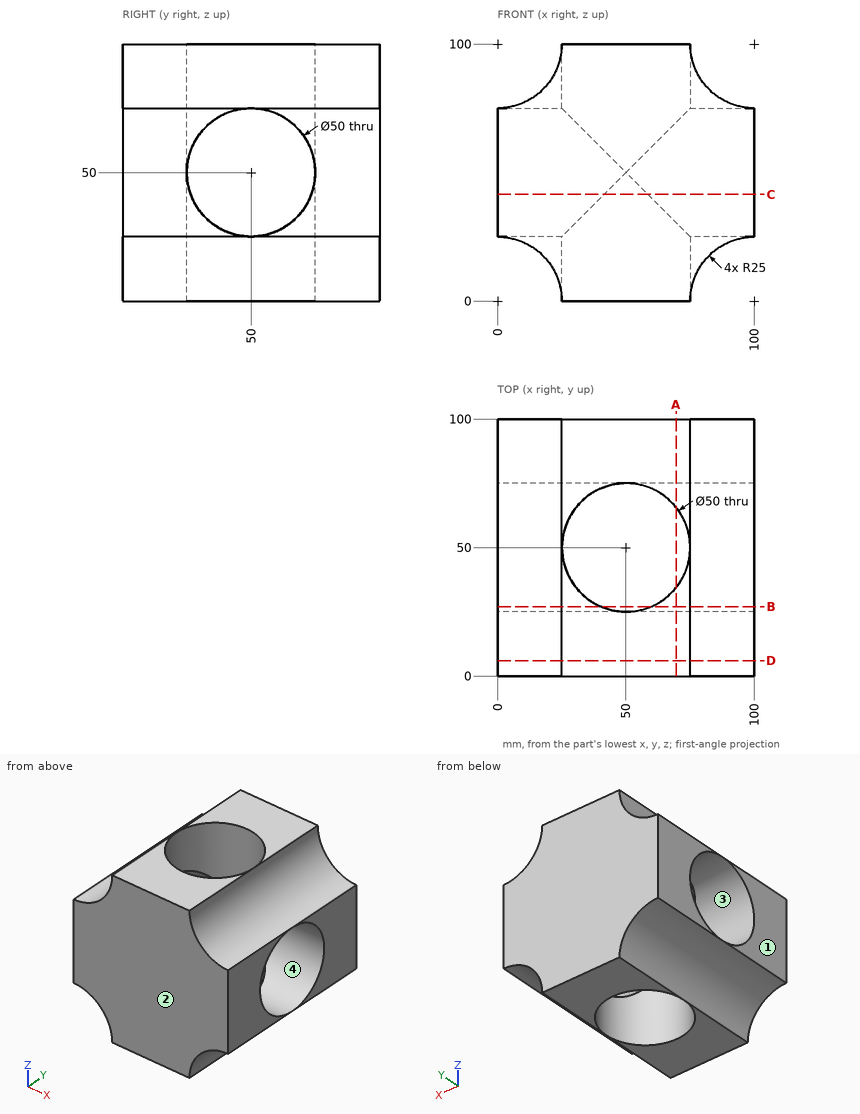
Here's the drawing with two shaded views (mm, measured from the low corner). I have some questions. Give positions to 0.01 mm unless a question says otherwise; leave off trailing zeros. Loops run counter-clockwise (first coordinate to the right, second up) from the corner with the lowest first, then second, coordinate; pieces in that order, holes last. Notation, with made-up numbers: (25.25, 73) -> (81.25, 73) arc R30 ccw to (81.25, 99) -> close; hole circle Ø4 at (72.5, -19.5). An arc over 180 degrees is marked (long way). Answer as a JSON object with one key per item and string values. Group by question number.
Item 1: Imagine slicing it at B-B on y = 27. Write out the boundary of the cut face in (x, z), then the cut area to 3 significant figures.
Item 2: Imagine slicing it at D-D on y = 6. Write out the boundary of the cut face in (x, z), then the cut area to 3 significant figures.
Item 3: Imagine slicing it at C-C on z = 41.5. Write out the boundary of the cut face in (x, y).
Item 4: Thinking about a two-plate mould opening in Y: for the marked faces 1, 2, 3 and 4, which applies, pulls with the +Y half, pulls with the -Y half, needs draft (parallel to the pull), parting line crosses it, or undercut?
Item 5: Imagine slicing it at A-A on x = 69.5. Write out the boundary of the cut face in (y, z), then the cut area to 3 significant figures.
Item 6: Will these pins go through, and if not, where does the flat tip stop? pin 1 (1 mm diameter, centred on x = 14.5, y = 30, fed in from +Z); pin 2 (8 mm diameter, centred on y = 71, z = 87.5, fed in from -X); pin 3 (1.5 mm diameter, centred on x = 13, y = 15.5, fed in from +Z).
Item 7: I need wall thicknesses on L1, parallel to Y at x = 13, z = 50; L2, parallel to Y at x = 77.5, z = 32.5; L3, parallel to X at y = 55, z = 78. Which ranges of each line are inside material? Lowest first, please.
Answer list:
{
 "1": {"outline": "(0, 25) arc R25 cw to (25, 0) -> (40.2, 0) -> (40.2, 40.2) -> (0, 40.2) -> close; (0, 59.8) -> (40.2, 59.8) -> (40.2, 100) -> (25, 100) arc R25 cw to (0, 75) -> close; (59.8, 0) -> (75, 0) arc R25 cw to (100, 25) -> (100, 40.2) -> (59.8, 40.2) -> close; (59.8, 59.8) -> (100, 59.8) -> (100, 75) arc R25 cw to (75, 100) -> (59.8, 100) -> close", "area": "4,500 mm2"},
 "2": {"outline": "(0, 25) arc R25 cw to (25, 0) -> (75, 0) arc R25 cw to (100, 25) -> (100, 75) arc R25 cw to (75, 100) -> (25, 100) arc R25 cw to (0, 75) -> close", "area": "8,040 mm2"},
 "3": {"outline": "(0, 0) -> (100, 0) -> (100, 26.49) -> (58.5, 26.49) arc R25 cw to (41.5, 26.49) -> (0, 26.49) -> close; (0, 73.51) -> (41.5, 73.51) arc R25 cw to (58.5, 73.51) -> (100, 73.51) -> (100, 100) -> (0, 100) -> close"},
 "4": {"face 1": "needs draft", "face 2": "pulls with the -Y half", "face 3": "undercut", "face 4": "undercut"},
 "5": {"outline": "(0, 0) -> (34.36, 0) -> (34.36, 30.5) arc R25 cw to (34.36, 69.5) -> (34.36, 100) -> (0, 100) -> close; (65.64, 0) -> (100, 0) -> (100, 100) -> (65.64, 100) -> (65.64, 69.5) arc R25 cw to (65.64, 30.5) -> close", "area": "6,360 mm2"},
 "6": {"pin 1": "stops at z = 80", "pin 2": "stops at x = 18.78", "pin 3": "stops at z = 79.12"},
 "7": {"L1": "y = 0 to 25, 75 to 100", "L2": "y = 0 to 32.15, 67.85 to 100", "L3": "x = 11.87 to 25.51, 74.49 to 88.13"}
}
